Input: dimensioned drawing with shaded views. Units: mm. Origin: part minimum x, y, z. A direction names the side the tool comes from. Give positions to 0.01 mm unless a question says otherwise; leave off trailing zeros. Loops run counter-clockwise (first coordinate to the right, second up) from the corner with the lowest first, then second, coordinate; pieces in that order, holes last. Notation, with made-up numbers: M 59.5,45 L 106.5,45 A25 ccw 106.5,81 Z; hole C 83,59 d7. An arc over 180 degrees is marked long. Use CSV: the item, a comma, the result in double quotes. Start each with the question number.
Q1. Section A-A, the plane x = 315. Output: boundary loops of the cut face in (y, z), plus the area to 3 significant figures.
Q2. Section D-D, the plane z = 719. Output: boundary loops of the cut face in (x, y), plus the area to 3 significant figures.
Q3. Section C-C, the plane y = 109. Output: boundary loops of the cut face in (x, z), plus the area to 3 significant figures.
Q4. Material intervals for line 1 along X through (y, z) = (136, 719.5); line 2 along Y through (x, z) = (362, 848); line 3 along Y through (x, z) = (133.5, 107), sorted ascending.
Q5. Pull-direction query (Y, two-part tool) for the marked faces 1, 2, 3 and 4; classes: released by +Y, released by -Y, zero draft, split by the parting line, or undercut.
Q6. Reachability of the marked faces 5, 6 and 7 from +Z, -Z, +X, -X, +Y, -Y: full face, straight path, thin tool, end or side. Return the list, or none.
Q7. Pin query (flat end, axial travel): pin 1 (12 mm diameter, centred on x = 104.5, y = 134, fed in from -Z); pin 2 (8 mm diameter, centred on y = 124.5, z = 783.5, fed in from +X) (1 decimal); pin 3 (1 mm diameter, centred on y = 110, z = 588, fed in from +X). Return the tip coordinate at first contact, or that it passes through.
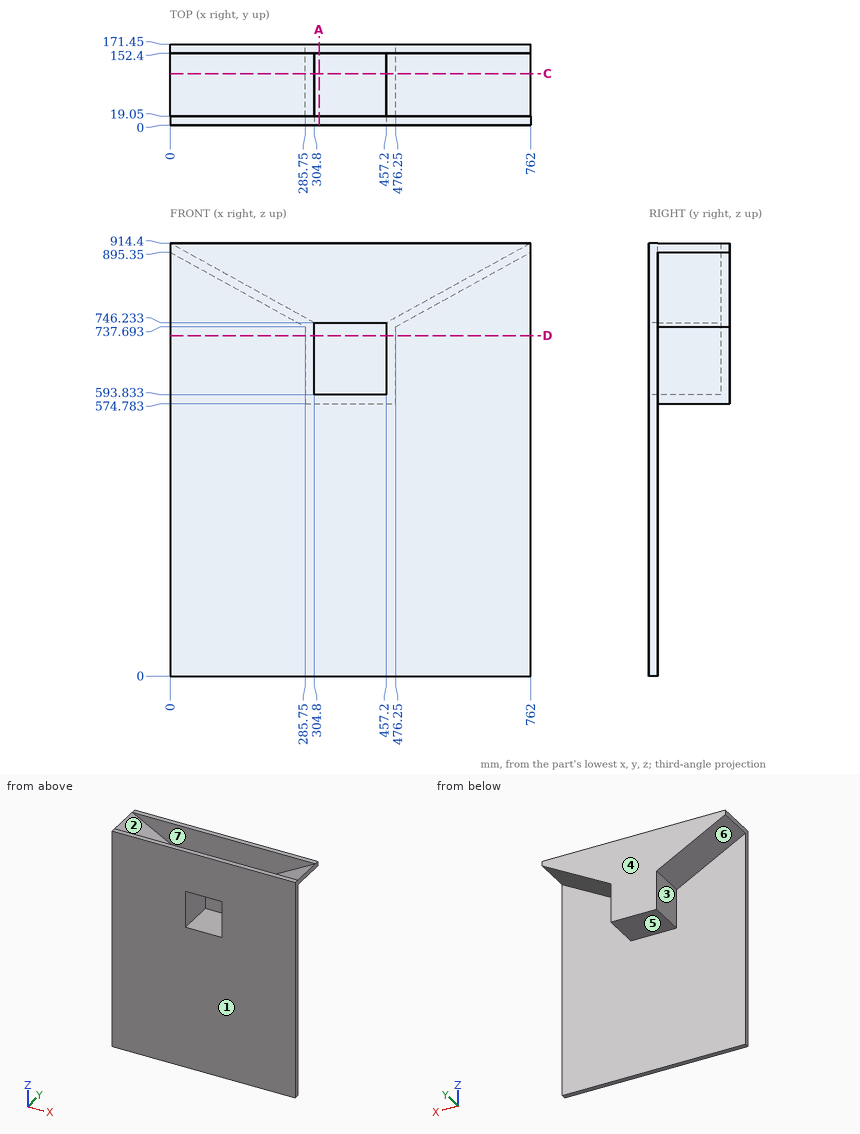
A:
1,outline,"M 0,0 L 19.05,0 L 19.05,574.78 L 171.45,574.78 L 171.45,914.4 L 152.4,914.4 L 152.4,593.83 L 0,593.83 Z; M 0,746.23 L 19.05,746.23 L 19.05,914.4 L 0,914.4 Z"
1,area,"23,500 mm^2"
2,outline,"M 0,0 L 304.8,0 L 304.8,152.4 L 457.2,152.4 L 457.2,0 L 762,0 L 762,19.05 L 476.25,19.05 L 476.25,171.45 L 285.75,171.45 L 285.75,19.05 L 0,19.05 Z"
2,area,"20,300 mm^2"
3,outline,"M 0,895.35 L 285.75,737.69 L 285.75,574.78 L 476.25,574.78 L 476.25,737.69 L 762,895.35 L 762,914.4 L 457.2,746.23 L 457.2,593.83 L 304.8,593.83 L 304.8,746.23 L 0,914.4 Z"
3,area,"20,500 mm^2"
4,line 1,"285.75 to 304.8, 457.2 to 476.25"
4,line 2,"0 to 19.05, 152.4 to 171.45"
4,line 3,"0 to 19.05"
5,face 1,"released by -Y"
5,face 2,"undercut"
5,face 3,"zero draft"
5,face 4,"released by +Y"
6,face 5,"-Z, +X, -X, +Y"
6,face 6,"-Z, -X, +Y"
6,face 7,"+Z"
7,pin 1,"z = 834.38"
7,pin 2,"x = 566.5"
7,pin 3,"x = 476.25"
